Build history of the part. All positions in model axes, mm. Round coordinates to 2 decimals unless told otherwise and drop trailing zeros. Order: outer loops, then holes, each group sorted by start corner. A loop starts at its lowest first (then second) coordinate and runs counter-clockwise, first axis right, second up. Notation, with made-up numbers: M 77,-23 L 125,-23 A20 cw 125,-5 Z; hole C 24.5,-12 d3. An arc over 180 degrees is marked long. One line per item, written item: value. Start each with the question number.
Item 1: Probe L1, parallel to Z at x = 0.2, y = 27; L2, parallel to Y at x = -0.1, z = 21; L3, parallel to Y at x = 0.9, z = 6. List the from-to ranges inside material, lowest first.
Item 2: Pin check, flat tips, straight feed: pin 1 (0.8 mm diameter, centred on x = 0, z = 5, fed in from +Y); pin 2 (1.1 mm diameter, centred on y = 23.5, z = 65.5, fed in from +X); pin 3 (0.5 mm diameter, centred on y = 35, z = 65.5, fed in from -X). Stop position of each tip, or through.
Item 3: Band-saw the part on B-B, the plane z = 12.5. Write the cut outline in (x, y).
Item 4: Two-plate mould, pull along Z, no slides. Class faces 1 (the flat face through (0, 1.48, 4)), 2 (the flat face through (0, 19, 65.8)), 3 (the flat face through (0, 0, 0)): +Z half, -Z half, draft (parallel to the pull), parting line (faces both ways), or undercut.
Item 5: Band-saw the part on A-A, the plane y = 20. Write the cut outline in (x, z).
```python
from build123d import *

# Parameters (mm, degrees)
SKETCH1_R           = 2
BOSS_EXTRUDE1_DEPTH = 65.8
CUT_EXTRUDE1_DEPTH  = 8
SKETCH3_W           = 1
SKETCH3_H           = 50
BOSS_EXTRUDE2_DEPTH = 1


with BuildPart() as part:
    # Sketch1 → Boss-Extrude1 (new body)
    with BuildSketch(Plane.XY):
        Circle(SKETCH1_R)
    extrude(amount=BOSS_EXTRUDE1_DEPTH)

    # Sketch2 → Cut-Extrude1 (cut)
    with BuildSketch(Plane(origin=(0, 0, 0), x_dir=(-1, 0, 0), z_dir=(0, 0, -1))):
        with BuildLine():
            Line((-1.345213738, 1.48), (1.345213738, 1.48))
            ThreePointArc((1.345213738, 1.48), (0, 2), (-1.345213738, 1.48))
        make_face()
    extrude(amount=-CUT_EXTRUDE1_DEPTH, mode=Mode.SUBTRACT)

    # Sketch3 → Boss-Extrude2 (add)
    with BuildSketch(Plane.XY.offset(65.8)):
        with Locations((0, 25)):
            Rectangle(SKETCH3_W, SKETCH3_H)
    extrude(amount=-BOSS_EXTRUDE2_DEPTH)


solid = part.part
```
Output:
1. L1: z = 64.8 to 65.8
1. L2: y = -2 to 2
1. L3: y = -1.79 to 1.48
2. pin 1: stops at y = 1.48
2. pin 2: stops at x = 0.5
2. pin 3: stops at x = -0.5
3. outline: C 0,0 d4
4. face 1: draft
4. face 2: +Z half
4. face 3: -Z half
5. outline: M -0.5,64.8 L 0.5,64.8 L 0.5,65.8 L -0.5,65.8 Z
